Design review of the part shown in the three views and the two pictorial views. Dimensions are in mm from the part's minimum x, y and z. Give positions to 0.01 mm unless a question says otherwise; leave off trailing zeros. Order: outer loops, then holes, each group sorted by start corner. A loop starts at its lowest first (then second) coordinate and runs counter-clockwise, first axis right, second up.
Item 1: For P1, Ø11.5, axis at x = 123, z = 171, coming from the -Y side; P2, Ø10, axis at x = 225.5, y = 26.5, coming from the -Z side; P3, Ø6, axis at x = 119, y = 21, coming from the +Z side, all flat-tipped, find the tip position at first contact; note any pin that passes through.
Item 2: Consider section B-B (y = 8.5). Give the boundary of the cut face in (x, z), plus the area to 3 significant figures.
Item 3: Consider section A-A (z = 171.45). Give the boundary of the cut face in (x, y).
Item 4: Consider section C-C (z = 120.65). Give the boundary of the cut face in (x, y), plus the area to 3 significant figures.
Item 5: Consider section D-D (x = 226). Give the boundary of the cut face in (y, z).
Item 6: For probe 1 along X at (y, z) = (11, 171); probe 2 along X at (y, z) = (9.5, 182.5), list the stretches that pass through material, from the lowest coordinate up.
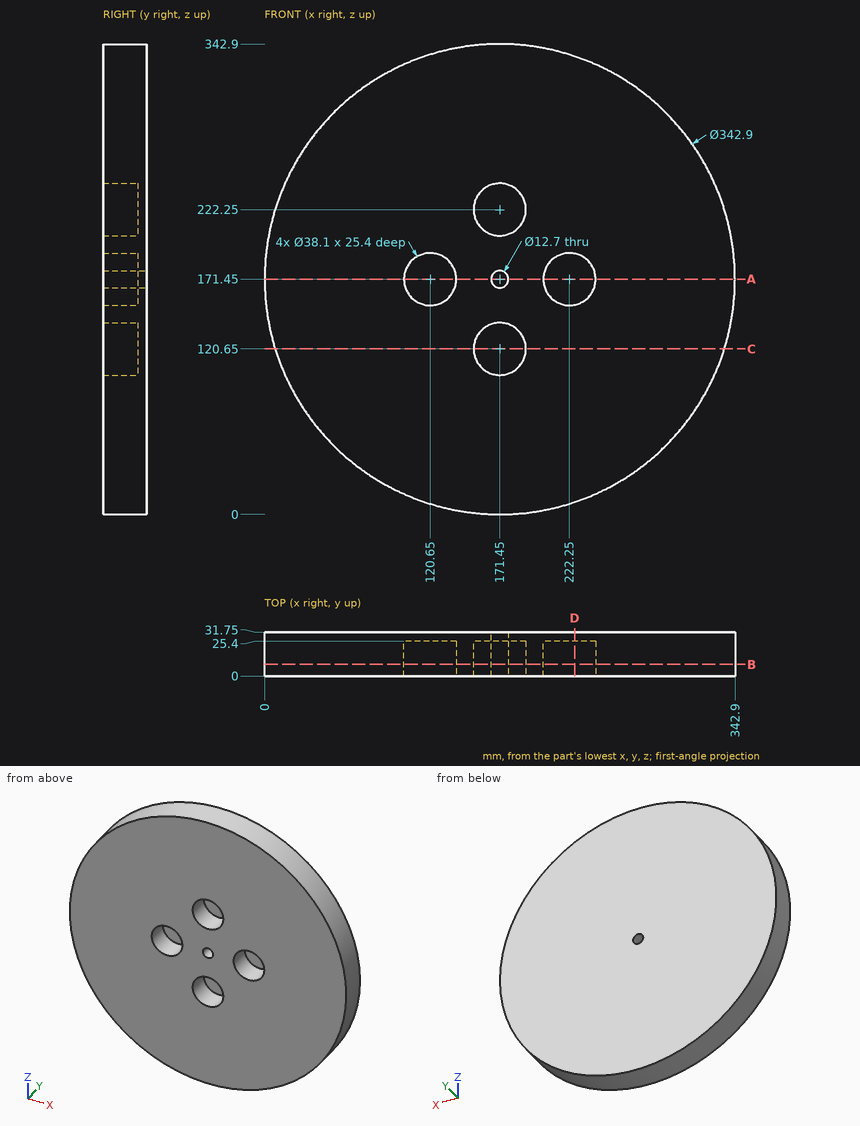
Resolved:
1. P1: stops at y = 25.4
1. P2: stops at z = 7.17
1. P3: stops at z = 335.61
2. outline: circle Ø342.9 at (171.45, 171.45); hole circle Ø38.1 at (120.65, 171.45); hole circle Ø38.1 at (171.45, 120.65); hole circle Ø38.1 at (171.45, 222.25); hole circle Ø12.7 at (171.45, 171.45); hole circle Ø38.1 at (222.25, 171.45)
2. area: 87,700 mm2
3. outline: (0, 0) - (101.6, 0) - (101.6, 25.4) - (139.7, 25.4) - (139.7, 0) - (165.1, 0) - (165.1, 31.75) - (0, 31.75) - close; (177.8, 0) - (203.2, 0) - (203.2, 25.4) - (241.3, 25.4) - (241.3, 0) - (342.9, 0) - (342.9, 31.75) - (177.8, 31.75) - close
4. outline: (7.7, 0) - (152.4, 0) - (152.4, 25.4) - (190.5, 25.4) - (190.5, 0) - (335.2, 0) - (335.2, 31.75) - (7.7, 31.75) - close
4. area: 9,430 mm2
5. outline: (0, 8.91) - (31.75, 8.91) - (31.75, 333.99) - (0, 333.99) - (0, 190.13) - (25.4, 190.13) - (25.4, 152.77) - (0, 152.77) - close
6. probe 1: x = 0 to 101.61, 139.69 to 165.12, 177.78 to 203.21, 241.29 to 342.9
6. probe 2: x = 0.36 to 105.13, 136.17 to 206.73, 237.77 to 342.54
